Source: three-view drawing plus pictorial views. Frame: mm from the lowest corner of the part. A direction names the side the tool comes from. Give positions to 0.01 mm unless a question says otherwise; leave off trailing zeros. Write each loop counter-clockwise with the first axis right and the second up, starting at its lowest first coordinate (ties: lowest second). Pieces come first, ordered by that corner, then holes.
Q1. Cut plane A-A on y = 7. Return the cut outline in (x, z).
Q2. Line query: L1, parallel to Z at x = 6.25, y = 15.25; L2, parallel to X at y = 7.25, z = 2; L3, parallel to Y at x = 13.5, z = 0.6. Output: solid intervals per line, ascending.
Q3. Reachability of the marked faces 1 and 2 from +Z, -Z, +X, -X, +Y, -Y: full face, straight path, thin tool, end or side. Return the list, or none.
Q4. Draft query along Y for the marked faces 3, 4 and 5. Return one class per face: pulls with the +Y half, pulls with the -Y half, needs draft (parallel to the pull), parting line crosses it, or undercut.
Q5. Pin query (flat end, axial travel): pin 1 (1.6 mm diameter, centred on x = 1.5, y = 7, fed in from +Z); pin 2 (1.6 mm diameter, centred on y = 8, z = 2.5, fed in from +X); pin 3 (1.6 mm diameter, centred on y = 7.5, z = 2.5, fed in from -X); pin 4 (0.8 mm diameter, centred on x = 8.5, z = 2.5, fed in from +Y). Return the tip coordinate at first contact, or that it passes through.
Q6. Cut plane C-C on x = 1.5. Return the cut outline in (y, z).
Q7. Cut plane D-D on z = 2.2. Return the cut outline in (x, y).
Q8. Cut plane B-B on z = 1.3. Return the cut outline in (x, y), plus the area to 3 significant figures.
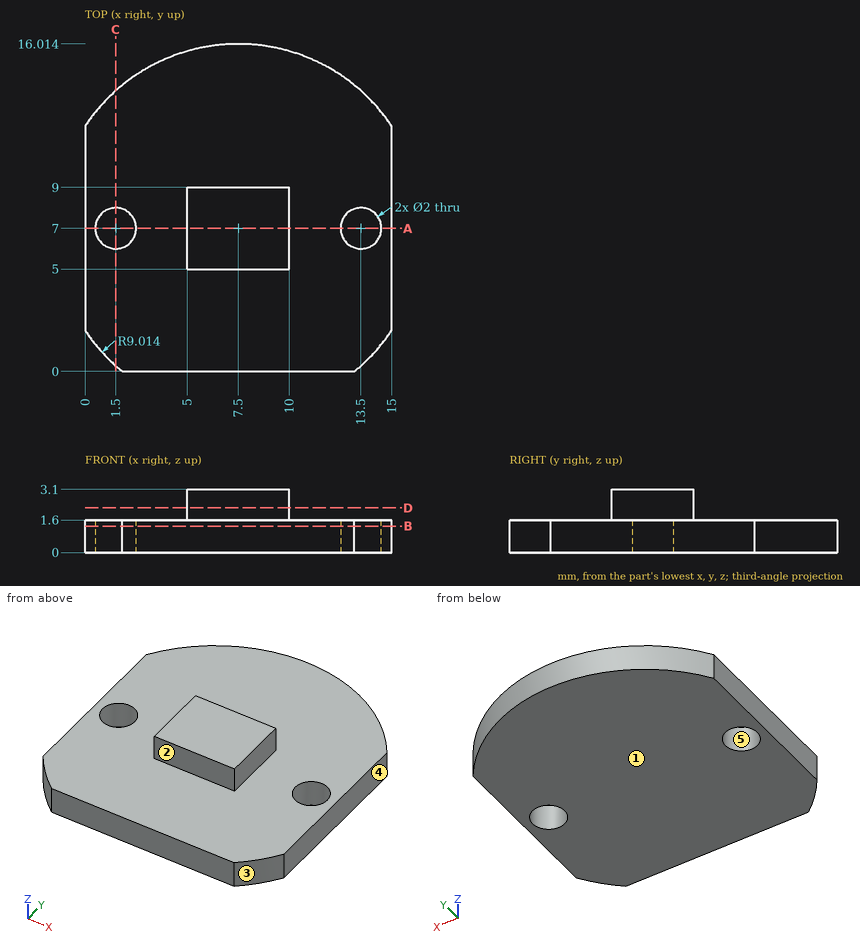
Data:
1. outline: (0, 0) - (0.5, 0) - (0.5, 1.6) - (0, 1.6) - close; (2.5, 0) - (12.5, 0) - (12.5, 1.6) - (10, 1.6) - (10, 3.1) - (5, 3.1) - (5, 1.6) - (2.5, 1.6) - close; (14.5, 0) - (15, 0) - (15, 1.6) - (14.5, 1.6) - close
2. L1: z = 0 to 1.6
2. L2: x = 5 to 10
2. L3: y = 0.27 to 6, 8 to 13.73
3. face 1: -Z, +X, -X, +Y, -Y
3. face 2: +Z, +X, -X, -Y
4. face 3: pulls with the -Y half
4. face 4: needs draft
4. face 5: undercut
5. pin 1: passes through
5. pin 2: stops at x = 10
5. pin 3: stops at x = 5
5. pin 4: stops at y = 9
6. outline: (0.27, 0) - (6, 0) - (6, 1.6) - (0.27, 1.6) - close; (8, 0) - (13.73, 0) - (13.73, 1.6) - (8, 1.6) - close
7. outline: (5, 5) - (10, 5) - (10, 9) - (5, 9) - close
8. outline: (0, 2) arc R9.01 ccw to (1.82, 0) - (13.18, 0) arc R9.01 ccw to (15, 2) - (15, 12) arc R9.01 ccw to (0, 12) - close; hole circle Ø2 at (1.5, 7); hole circle Ø2 at (13.5, 7)
8. area: 213 mm2
